from build123d import *

# Parameters (mm, degrees)
SKETCH6_W            = 62.23
SKETCH6_H            = 2.032
BOSS_EXTRUDE2_DEPTH  = 3.175
BOSS_EXTRUDE3_DEPTH  = 3.175
LPATTERN2_COUNT      = 24
LPATTERN2_PITCH      = 2.493518
SKETCH9_W            = 2.910078
SKETCH9_H            = 2.032
CUT_EXTRUDE1_DEPTH   = 3.175
SKETCH10_W           = 59.319922
SKETCH10_H           = 6.35
BOSS_EXTRUDE4_DEPTH  = 0.508
SKETCH11_W           = 68.58
SKETCH11_H           = 2.54
BOSS_EXTRUDE5_DEPTH  = 6.35
SKETCH12_W           = 6.35
SKETCH12_H           = 6.35
BOSS_EXTRUDE6_DEPTH  = 1.778
SKETCH14_W           = 31.115
SKETCH14_H           = 1.778
BOSS_EXTRUDE7_DEPTH  = 6.35
CUT_EXTRUDE2_REACH   = 66.378
SKETCH13_R           = 1.627
FILLET1_R            = 3.048
FILLET1_OF_MIRROR4_R = 3.048
CUT_EXTRUDE3_REACH   = 66.319
SKETCH16_W           = 5.94905084
SKETCH16_H           = 3.175
CUT_EXTRUDE4_REACH   = 66.241
SKETCH18_W           = 74.285931649
SKETCH18_H           = 23.332469726
SKETCH19_W           = 3.175
SKETCH19_H           = 6.1039375
CUT_EXTRUDE5_DEPTH   = 2.54
SKETCH20_W           = 3.175
SKETCH20_H           = 6.1039375
CUT_EXTRUDE6_DEPTH   = 2.54


with BuildPart() as part:
    # Sketch6 → Boss-Extrude2 (new, symmetric)
    with BuildSketch(Plane.XY):
        with Locations((31.115, 1.016)):
            Rectangle(SKETCH6_W, SKETCH6_H)
    extrude(amount=BOSS_EXTRUDE2_DEPTH, both=True)

    # Sketch7 → Boss-Extrude3 (add, symmetric)
    with BuildSketch(Plane.XY):
        Polygon((1.31901184, 3.8179375), (1.969008, 2.032), (0, 2.032), (0.64999616, 3.8179375), align=None)
    boss_extrude3 = extrude(amount=BOSS_EXTRUDE3_DEPTH, both=True)

    # LPattern2: Boss-Extrude3 ×24
    with Locations(*[(i * LPATTERN2_PITCH, 0, 0) for i in range(1, LPATTERN2_COUNT)]):
        add(boss_extrude3)

    # Sketch9 → Cut-Extrude1 (cut, symmetric)
    with BuildSketch(Plane.XY):
        with Locations((60.774961, 1.016)):
            Rectangle(SKETCH9_W, SKETCH9_H)
    extrude(amount=CUT_EXTRUDE1_DEPTH, both=True, mode=Mode.SUBTRACT)

    # Sketch10 → Boss-Extrude4 (add)
    with BuildSketch(Plane.XZ):
        with Locations((29.659961, 0)):
            Rectangle(SKETCH10_W, SKETCH10_H)
    extrude(amount=BOSS_EXTRUDE4_DEPTH)

    # Sketch11 → Boss-Extrude5 (add)
    with BuildSketch(Plane.XY.offset(3.175)):
        with Locations((29.659961, 0.762)):
            Rectangle(SKETCH11_W, SKETCH11_H)
    extrude(amount=-BOSS_EXTRUDE5_DEPTH)

    # Sketch12 → Boss-Extrude6 (add)
    with BuildSketch(Plane.XZ.offset(0.508)):
        with Locations((-1.455039, 0)):
            Rectangle(SKETCH12_W, SKETCH12_H)
    boss_extrude6 = extrude(amount=BOSS_EXTRUDE6_DEPTH)

    # Sketch14 → Boss-Extrude7 (add)
    with BuildSketch(Plane.XY.offset(3.175)):
        Polygon((-4.630039, 2.92496875), (-4.630039, 2.032), (0, 2.032), (0.32499808, 2.92496875), (0.64999616, 3.8179375), (-4.630039, 3.8179375), align=None)
        with Locations((17.277461, -1.397)):
            Rectangle(SKETCH14_W, SKETCH14_H)
    boss_extrude7 = extrude(amount=-BOSS_EXTRUDE7_DEPTH)

    # Sketch13 → Cut-Extrude2 (cut, up to next)
    with BuildSketch(Plane.XY.offset(3.175), mode=Mode.PRIVATE) as cut_extrude2_sk1:
        with Locations((-1.455039, 0.762)):
            Circle(SKETCH13_R)
    cut_extrude2_tool1 = extrude(cut_extrude2_sk1.sketch, amount=-CUT_EXTRUDE2_REACH, mode=Mode.PRIVATE) & part.part
    cut_extrude2 = cut_extrude2_tool1.solids().sort_by_distance((-1.455039, 0.762, 3.175))[0]
    add(cut_extrude2, mode=Mode.SUBTRACT)

    # Fillet1
    fillet1_edges = [part.edges().sort_by_distance(p)[0] for p in [
        (-4.630039, -2.286, 0),
        (-4.630039, 3.8179375, 0),
    ]]
    fillet(fillet1_edges, radius=FILLET1_R)

    # Mirror4: Boss-Extrude6, Boss-Extrude7, Cut-Extrude2 across plane
    add(boss_extrude6.mirror(Plane.ZY.offset(-29.659961)))
    add(boss_extrude7.mirror(Plane.ZY.offset(-29.659961)))
    add(cut_extrude2.mirror(Plane.ZY.offset(-29.659961)), mode=Mode.SUBTRACT)

    # Fillet1 of Mirror4
    fillet1_of_mirror4_edges = [part.edges().sort_by_distance(p)[0] for p in [
        (63.949961, -2.286, 0),
        (63.949961, 3.8179375, 0),
    ]]
    fillet(fillet1_of_mirror4_edges, radius=FILLET1_OF_MIRROR4_R)

    # Sketch16 → Cut-Extrude3 (cut, up to next)
    with BuildSketch(Plane(origin=(0, 3.8179375, 0), x_dir=(1, 0, 0), z_dir=(0, 1, 0)), mode=Mode.PRIVATE) as cut_extrude3_sk1:
        with Locations((-1.65551358, -1.5875)):
            Rectangle(SKETCH16_W, SKETCH16_H)
    cut_extrude3_tool1 = extrude(cut_extrude3_sk1.sketch, amount=-CUT_EXTRUDE3_REACH, mode=Mode.PRIVATE) & part.part
    # Sketch16 → Cut-Extrude3 (cut, up to next)
    with BuildSketch(Plane(origin=(0, 3.8179375, 0), x_dir=(1, 0, 0), z_dir=(0, 1, 0)), mode=Mode.PRIVATE) as cut_extrude3_sk2:
        with Locations((60.97543558, -1.5875)):
            Rectangle(SKETCH16_W, SKETCH16_H)
    cut_extrude3_tool2 = extrude(cut_extrude3_sk2.sketch, amount=-CUT_EXTRUDE3_REACH, mode=Mode.PRIVATE) & part.part
    add(cut_extrude3_tool1.solids().sort_by_distance((-1.655514, 3.817937, 1.5875))[0], mode=Mode.SUBTRACT)
    add(cut_extrude3_tool2.solids().sort_by_distance((60.975436, 3.817937, 1.5875))[0], mode=Mode.SUBTRACT)

    # Sketch18 → Cut-Extrude4 (cut, up to next)
    with BuildSketch(Plane.XY.offset(1.5875), mode=Mode.PRIVATE) as cut_extrude4_sk1:
        with Locations((31.985939291, 1.965301306)):
            Rectangle(SKETCH18_W, SKETCH18_H)
    cut_extrude4_tool1 = extrude(cut_extrude4_sk1.sketch, amount=CUT_EXTRUDE4_REACH, mode=Mode.PRIVATE) & part.part
    add(cut_extrude4_tool1.solids().sort_by_distance((31.985939, 1.965301, 1.5875))[0], mode=Mode.SUBTRACT)

    # Mirror11: part across plane


with BuildPart() as part_1:
    add(part.part)
    add(part.part.mirror(Plane.XY.offset(1.5875)))

    # Sketch19 → Cut-Extrude5 (cut)
    with BuildSketch(Plane(origin=(58.00091016, 0, 0), x_dir=(0, 0, -1), z_dir=(1, 0, 0))):
        with Locations((-1.5875, 0.76596875)):
            Rectangle(SKETCH19_W, SKETCH19_H)
    extrude(amount=-CUT_EXTRUDE5_DEPTH, mode=Mode.SUBTRACT)

    # Sketch20 → Cut-Extrude6 (cut)
    with BuildSketch(Plane.ZY.offset(-1.31901184)):
        with Locations((1.5875, 0.76596875)):
            Rectangle(SKETCH20_W, SKETCH20_H)
    extrude(amount=-CUT_EXTRUDE6_DEPTH, mode=Mode.SUBTRACT)


solid = part_1.part
For this review, take the finished solid that the model builds, in its own axes (mm). A direction names the side the tool comes from. Round coordinates to 2 decimals unless told otherwise and drop trailing zeros. Loops run counter-clockwise (first coordinate to the right, second up) from the corner with the lowest first, then second, coordinate; pieces in that order, holes last. Notation, with made-up numbers: (28, 32.25) - (49, 32.25) arc R18 ccw to (49, 43.25) - close; hole circle Ø10 at (75.25, 52). An arc over 180 degrees is marked (long way). Use one line per item in the form item = value.
1) Wall thickness on probe 1 along Z at (x, y) = (56, -0.75) (3 decimals); probe 2 along X at (y, z) = (1.5, 4.25); probe 3 along X at (y, z) = (-1, 3): over which ranges is each line inside the solid? List them lowest first.
Solutions:
probe_1 = -3.175 to 0, 3.175 to 6.35
probe_2 = -4.54 to -2.91, -0.01 to 59.32, 62.22 to 63.86
probe_3 = 3.86 to 55.46
2) Clearance check with flat-ended pins moving along their axes: P1, Ø2, axis at y = 3, z = -1, coming from the -X side; P2, Ø1, axis at y = 3, z = 2, coming from the -X side. State where each tip first meets the part, or that it passes through.
Solutions:
P1 = -4.37
P2 = 3.86
3) Tool access review of faces 1 (the face through (61.974, 1.862, 4.74)), 2 (the face through (59, 1, 0)), 3 (the face through (27.75, 2.91, 1.52)): name each direction out of +Z, -Z, +X, -X, +Y, -Y from which nothing blocks a thin tool from reaching the whole face with its end or side.
Solutions:
face_1 = +Z, -Z
face_2 = +X, +Y, -Y
face_3 = +Z, -Z, +Y
4) Mouldability with a two-part tool opening along Y and no side actions: class faces 4 (the face through (47.697, 2.912, 1.521)), 5 (the face through (30, 0, 6.35)), 6 (the face through (-0.58, 2.134, 4.74)) as pulls with the +Y half, pulls with the -Y half, needs draft (parallel to the pull), parting line crosses it, or undercut.
Solutions:
face_4 = pulls with the +Y half
face_5 = needs draft
face_6 = undercut
5) We need section A-A on y = 0. Write out the cut boundary in (x, z) (3 decimals), then the cut area to 3 significant figures.
Solutions:
outline = (-4.533, -3.175) - (-2.893, -3.175) - (-2.893, 0) - (-4.533, 0) - close; (-4.533, 3.175) - (-2.893, 3.175) - (-2.893, 6.35) - (-4.533, 6.35) - close; (-0.018, -3.175) - (59.337, -3.175) - (59.337, 0) - (55.461, 0) - (55.461, 3.175) - (59.337, 3.175) - (59.337, 6.35) - (-0.018, 6.35) - (-0.018, 3.175) - (3.859, 3.175) - (3.859, 0) - (-0.018, 0) - close; (62.212, -3.175) - (63.853, -3.175) - (63.853, 0) - (62.212, 0) - close; (62.212, 3.175) - (63.853, 3.175) - (63.853, 6.35) - (62.212, 6.35) - close
area = 562 mm2
6) We need section B-B on z = 5.5. State how many separate pieces and enclosed holes the cut face has, then the cut area to 3 significant figures.
Solutions:
separate_pieces = 1
enclosed_holes = 2
area = 346 mm2
